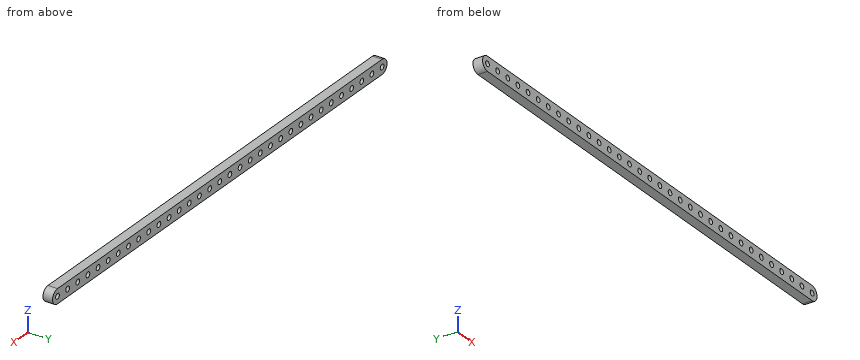
from build123d import *

# Parameters (mm, degrees)
SKETCH1_R           = 1.778
BOSS_EXTRUDE1_DEPTH = 6.35


with BuildPart() as part:
    # Sketch1 → Boss-Extrude1 (new body)
    with BuildSketch(Plane(origin=(0, 6.35, 0), x_dir=(1, 0, 0), z_dir=(0, 1, 0))):
        with BuildLine():
            Line((156.464, 4.7625), (-156.464, 4.7625))
            ThreePointArc((-156.464, 4.7625), (-161.2265, 0), (-156.464, -4.7625))
            Line((-156.464, -4.7625), (156.464, -4.7625))
            ThreePointArc((156.464, -4.7625), (161.2265, 0), (156.464, 4.7625))
        make_face()
        with Locations(Location((156.464, 0, 0), (0, 0, 270))):
            Circle(SKETCH1_R, mode=Mode.SUBTRACT)
        with Locations(Location((146.685, 0, 0), (0, 0, 270))):
            Circle(SKETCH1_R, mode=Mode.SUBTRACT)
        with Locations(Location((136.906, 0, 0), (0, 0, 270))):
            Circle(SKETCH1_R, mode=Mode.SUBTRACT)
        with Locations(Location((127.127, 0, 0), (0, 0, 270))):
            Circle(SKETCH1_R, mode=Mode.SUBTRACT)
        with Locations(Location((117.348, 0, 0), (0, 0, 270))):
            Circle(SKETCH1_R, mode=Mode.SUBTRACT)
        with Locations(Location((107.569, 0, 0), (0, 0, 270))):
            Circle(SKETCH1_R, mode=Mode.SUBTRACT)
        with Locations(Location((97.79, 0, 0), (0, 0, 270))):
            Circle(SKETCH1_R, mode=Mode.SUBTRACT)
        with Locations(Location((88.011, 0, 0), (0, 0, 270))):
            Circle(SKETCH1_R, mode=Mode.SUBTRACT)
        with Locations(Location((78.232, 0, 0), (0, 0, 270))):
            Circle(SKETCH1_R, mode=Mode.SUBTRACT)
        with Locations(Location((68.453, 0, 0), (0, 0, 270))):
            Circle(SKETCH1_R, mode=Mode.SUBTRACT)
        with Locations(Location((58.674, 0, 0), (0, 0, 270))):
            Circle(SKETCH1_R, mode=Mode.SUBTRACT)
        with Locations(Location((48.895, 0, 0), (0, 0, 270))):
            Circle(SKETCH1_R, mode=Mode.SUBTRACT)
        with Locations(Location((39.116, 0, 0), (0, 0, 270))):
            Circle(SKETCH1_R, mode=Mode.SUBTRACT)
        with Locations(Location((29.337, 0, 0), (0, 0, 270))):
            Circle(SKETCH1_R, mode=Mode.SUBTRACT)
        with Locations(Location((19.558, 0, 0), (0, 0, 270))):
            Circle(SKETCH1_R, mode=Mode.SUBTRACT)
        with Locations(Location((9.779, 0, 0), (0, 0, 270))):
            Circle(SKETCH1_R, mode=Mode.SUBTRACT)
        with Locations(Location((0, 0, 0), (0, 0, 270))):
            Circle(SKETCH1_R, mode=Mode.SUBTRACT)
        with Locations(Location((-9.779, 0, 0), (0, 0, 270))):
            Circle(SKETCH1_R, mode=Mode.SUBTRACT)
        with Locations(Location((-19.558, 0, 0), (0, 0, 270))):
            Circle(SKETCH1_R, mode=Mode.SUBTRACT)
        with Locations(Location((-29.337, 0, 0), (0, 0, 270))):
            Circle(SKETCH1_R, mode=Mode.SUBTRACT)
        with Locations(Location((-39.116, 0, 0), (0, 0, 270))):
            Circle(SKETCH1_R, mode=Mode.SUBTRACT)
        with Locations(Location((-48.895, 0, 0), (0, 0, 270))):
            Circle(SKETCH1_R, mode=Mode.SUBTRACT)
        with Locations(Location((-58.674, 0, 0), (0, 0, 270))):
            Circle(SKETCH1_R, mode=Mode.SUBTRACT)
        with Locations(Location((-68.453, 0, 0), (0, 0, 270))):
            Circle(SKETCH1_R, mode=Mode.SUBTRACT)
        with Locations(Location((-78.232, 0, 0), (0, 0, 270))):
            Circle(SKETCH1_R, mode=Mode.SUBTRACT)
        with Locations(Location((-88.011, 0, 0), (0, 0, 270))):
            Circle(SKETCH1_R, mode=Mode.SUBTRACT)
        with Locations(Location((-97.79, 0, 0), (0, 0, 270))):
            Circle(SKETCH1_R, mode=Mode.SUBTRACT)
        with Locations(Location((-107.569, 0, 0), (0, 0, 270))):
            Circle(SKETCH1_R, mode=Mode.SUBTRACT)
        with Locations(Location((-117.348, 0, 0), (0, 0, 270))):
            Circle(SKETCH1_R, mode=Mode.SUBTRACT)
        with Locations(Location((-127.127, 0, 0), (0, 0, 270))):
            Circle(SKETCH1_R, mode=Mode.SUBTRACT)
        with Locations(Location((-136.906, 0, 0), (0, 0, 270))):
            Circle(SKETCH1_R, mode=Mode.SUBTRACT)
        with Locations(Location((-146.685, 0, 0), (0, 0, 270))):
            Circle(SKETCH1_R, mode=Mode.SUBTRACT)
        with Locations(Location((-156.464, 0, 0), (0, 0, 270))):
            Circle(SKETCH1_R, mode=Mode.SUBTRACT)
    extrude(amount=-BOSS_EXTRUDE1_DEPTH)


solid = part.part
Geometry check sheet. Reference: the model listing, model coordinates, mm. Give positions to 0.01 mm unless a question says otherwise; leave off trailing zeros. Answer as CSV lines item,"result". Start each with the question number.
Q1. Material ranges on L1, parallel to Z at x = 117, y = 5; L2, parallel to Z at x = 97.79, y = 4.25; L3, parallel to X at y = 2, z = -4, recorded low to high.
Q2. Go/stop test with flat-tipped pins: pin 1 (2 mm diameter, centred on y = 4, z = -3, fed in from +X); pin 2 (3 mm diameter, centred on x = -136.906, z = 0, fed in from +Y); pin 3 (1.5 mm diameter, centred on y = 5, z = -2.5, fed in from +X). Record where each tip stops, or that it passes through.
Q3. Section check A-A, the plane z = 0. Give the number of separate pieces and of enclosed holes in the cut face, then the cut area to 3 significant figures.
Geometry says:
1,L1,"-4.76 to -1.74, 1.74 to 4.76"
1,L2,"-4.76 to -1.78, 1.78 to 4.76"
1,L3,"-159.05 to 159.05"
2,pin 1,"x = 160.79"
2,pin 2,"through"
2,pin 3,"x = 160.89"
3,separate pieces,"34"
3,enclosed holes,"0"
3,area,"1,300 mm^2"
